from build123d import *

# Parameters (mm, degrees)
BOSS_EXTRUDE1_DEPTH      = 25
BOSS_EXTRUDE1_DEPTH_BACK = 25
SKETCH1_R                = 15.875
SKETCH1_R_2              = 13.462
CUT_EXTRUDE1_DEPTH       = 25
CUT_EXTRUDE1_DEPTH_BACK  = 25
SKETCH2_R                = 2.5


with BuildPart() as part:
    # Sketch1 → Boss-Extrude1 (new, two sides: drawn at the far end of the back side and taken through both)
    with BuildSketch(Plane(origin=(0, 0, 0), x_dir=(0, 0, -1), z_dir=(1, 0, 0)).offset(-BOSS_EXTRUDE1_DEPTH_BACK)):
        Circle(SKETCH1_R)
        Circle(SKETCH1_R_2, mode=Mode.SUBTRACT)
    extrude(amount=BOSS_EXTRUDE1_DEPTH + BOSS_EXTRUDE1_DEPTH_BACK)

    # Sketch2 → Cut-Extrude1 (cut, two sides: drawn at the far end of the back side and taken through both)
    with BuildSketch(Plane.XY.offset(-CUT_EXTRUDE1_DEPTH_BACK)):
        with Locations(Location((-15, 0, 0), (0, 0, 180))):
            Circle(SKETCH2_R)
        with Locations(Location((15, 0, 0), (0, 0, 180))):
            Circle(SKETCH2_R)
    extrude(amount=CUT_EXTRUDE1_DEPTH + CUT_EXTRUDE1_DEPTH_BACK, mode=Mode.SUBTRACT)


solid = part.part
Part model, mm, in its own coordinate system. Coordinates: 2 decimals unless noted, no trailing zeros. Order: outer loops, then holes, each group sorted by start corner. A loop starts at its lowest first (then second) coordinate and runs counter-clockwise, first axis right, second up. Notation, with made-up numbers: M 42,19.25 L 62,19.25 A15 ccw 62,39.25 Z; hole C 89.5,62 d7. An arc over 180 degrees is marked long. Use a Markdown table: item, result.
(1) Cut at B-B on z = 0. Write the cut outline in (x, y) (3 decimals), then the cut area to 3 significant figures.
A:
| item | result |
|---|---|
| outline | M -25,-15.875 L 25,-15.875 L 25,-13.462 L -25,-13.462 Z; M -25,13.462 L 25,13.462 L 25,15.875 L -25,15.875 Z |
| area | 241 mm^2 |
(2) Cut at C-C on x = 15. Write the cut outline in (y, z) (3 decimals).
A:
| item | result |
|---|---|
| outline | M -2.5,-15.677 L -2.5,-13.228 A13.462 cw -2.5,13.228 L -2.5,15.677 A15.875 ccw Z; M 2.5,-15.677 A15.875 ccw 2.5,15.677 L 2.5,13.228 A13.462 cw 2.5,-13.228 Z |
(3) Cut at D-D on x = -10. Write the cut outline in (y, z) (3 decimals).
A:
| item | result |
|---|---|
| outline | C 0,0 d31.75; hole C 0,0 d26.924 |
(4) Pull direction Z, two halves, no side cores. Call faces 1 (the cylindrical face through (-0.35, -6.08, -14.664)), 2 (the flat face through (25, -12, 7)), 3 (the cylindrical face through (-0.35, -5.156, -12.435)): released by +Z, released by -Z, zero draft, split by the parting line, or undercut.
A:
| item | result |
|---|---|
| face 1 | split by the parting line |
| face 2 | zero draft |
| face 3 | undercut |
(5) Flat gauge pins, fed straight in: pin 1 (3 mm diameter, centred on x = 10.5, y = 2, fed in from -Z); pin 2 (1 mm diameter, centred on x = -7, y = 11.5, fed in from -Z); pin 3 (4 mm diameter, centred on x = 15, y = 0, fed in from -Z); pin 4 (2 mm diameter, centred on x = -4.5, z = 4, fed in from -Y). Where does each tip first touch, or does it go through?
A:
| item | result |
|---|---|
| pin 1 | stops at z = -15.87 |
| pin 2 | stops at z = -11.45 |
| pin 3 | passes through |
| pin 4 | stops at y = -15.59 |
(6) Cut at A-A on y = 0. Write the cut outline in (x, z) (3 decimals), then the cut area to 3 significant figures.
A:
| item | result |
|---|---|
| outline | M -25,-15.875 L -17.5,-15.875 L -17.5,-13.462 L -25,-13.462 Z; M -25,13.462 L -17.5,13.462 L -17.5,15.875 L -25,15.875 Z; M -12.5,-15.875 L 12.5,-15.875 L 12.5,-13.462 L -12.5,-13.462 Z; M -12.5,13.462 L 12.5,13.462 L 12.5,15.875 L -12.5,15.875 Z; M 17.5,-15.875 L 25,-15.875 L 25,-13.462 L 17.5,-13.462 Z; M 17.5,13.462 L 25,13.462 L 25,15.875 L 17.5,15.875 Z |
| area | 193 mm^2 |
(7) Probe L1, parallel to Y at x = -15, z = 0 (3 decimals); L2, parallel to Z at x = -7.5, y = -6.5; L3, parallel to Z at x = -16.5, y = 5. List the from-to ranges inside material, lowest first.
A:
| item | result |
|---|---|
| L1 | y = -15.875 to -13.462, 13.462 to 15.875 |
| L2 | z = -14.48 to -11.79, 11.79 to 14.48 |
| L3 | z = -15.07 to -12.5, 12.5 to 15.07 |
